```python
from build123d import *

# Parameters (mm, degrees)
F0_W     = 25
F0_H     = 70
F1_DEPTH = 5
F2_W     = 12
F2_H     = 4.5
F3_DEPTH = 14
F4_R     = 2
F5_R     = 5
F6_R     = 1


with BuildPart() as f1:
    # F0 (on Top) → F1 (new body, symmetric)
    with BuildSketch(Plane.XY):
        Rectangle(F0_W, F0_H)
    extrude(amount=F1_DEPTH, both=True)

    # F2 (on face) → F3 (join)
    with BuildSketch(Plane.XZ.offset(35)):
        Rectangle(F2_W, F2_H)
    extrude(amount=F3_DEPTH)

    # F4
    f4_edges = [f1.edges().sort_by_distance(p)[0] for p in [
        (12.5, -35, 0),
        (-12.5, -35, 0),
    ]]
    fillet(f4_edges, radius=F4_R)

    # F5
    f5_edges = [f1.edges().sort_by_distance(p)[0] for p in [
        (12.5, 35, 0),
        (-12.5, 35, 0),
    ]]
    fillet(f5_edges, radius=F5_R)

    # F6
    f6_edges = [f1.edges().sort_by_distance(p)[0] for p in [
        (-12.5, -1.5, 5),
        (-11.035534, 33.535534, 5),
        (-11.914214, -34.414214, 5),
        (0, 35, 5),
        (0, -35, 5),
        (11.035534, 33.535534, 5),
        (11.914214, -34.414214, 5),
        (12.5, -1.5, 5),
        (-12.5, -1.5, -5),
        (-11.035534, 33.535534, -5),
        (-11.914214, -34.414214, -5),
        (0, 35, -5),
        (0, -35, -5),
        (11.035534, 33.535534, -5),
        (11.914214, -34.414214, -5),
        (12.5, -1.5, -5),
    ]]
    fillet(f6_edges, radius=F6_R)


solid = f1.part
```
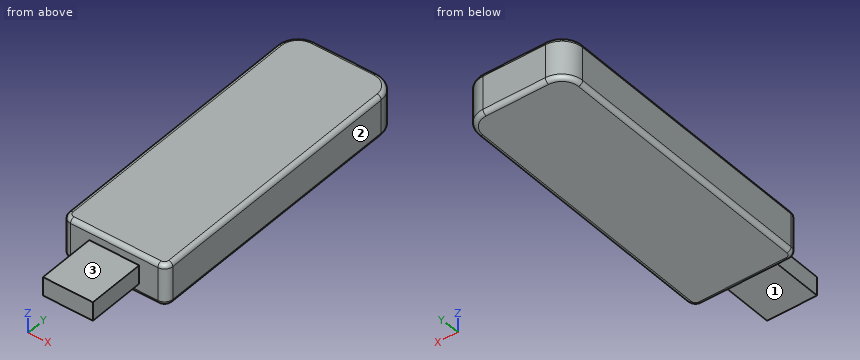
Check sheet for the modelled part. Datum: model origin and axes. Units: mm. Face numbers are marked on the shaded views. A direction names the side the tool comes from. Coordinates: 2 decimals unless noted, no trailing zeros. Loops run counter-clockwise (first coordinate to the right, second up) from the corner with the lowest first, then second, coordinate; pieces in that order, holes last. Notation, with made-up numbers: M -2,72.5 L 40,72.5 A27 ccw 40,101.5 Z; hole C 21,21 d9. An arc over 180 degrees is marked long. Answer as a JSON object with one key per item and string values.
1. Depth check by flat-ended pin: P1, Ø2, axis at y = -39.5, z = -0.5, coming from the +X side; P2, Ø13, axis at x = 2, y = -43, coming from the -Z side; P3, Ø6, axis at x = -1, y = -41, coming from the +Z side. Enter the tip coordinate at first touch or a pass-through.
Outcome:
{"P1": "x = 6", "P2": "z = -2.25", "P3": "z = 2.25"}
2. Access from +Z, -Z, +X, -X, +Y, -Y to the whole of each face (thin tool, end or side, straight path). Record for the marked faces 1, 2 and 3.
Outcome:
{"face 1": "-Z, +X, -X, -Y", "face 2": "+Z, -Z, +X, +Y, -Y", "face 3": "+Z, +X, -X, -Y"}
3. Scan lines: L1, parallel to Y at x = -6.5, z = 1.5; L2, parallel to Z at x = 2, y = -36.5; L3, parallel to X at y = -42.5, z = 1. Record each from-to range of solid material in increasing order. Write a range as from..to.
Outcome:
{"L1": "-35..35", "L2": "-2.25..2.25", "L3": "-6..6"}
4. Sectioned sample at A-A on x = 0. Record the cut outline in (y, z), and give its area (3 significant figures).
Outcome:
{"outline": "M -49,-2.25 L -35,-2.25 L -35,-4 A1 ccw -34,-5 L 34,-5 A1 ccw 35,-4 L 35,4 A1 ccw 34,5 L -34,5 A1 ccw -35,4 L -35,2.25 L -49,2.25 Z", "area": "762 mm²"}
5. Sectioned sample at B-B on z = 3.25. Record the cut outline in (x, y).
Outcome:
{"outline": "M -12.5,-33 A2 ccw -10.5,-35 L 10.5,-35 A2 ccw 12.5,-33 L 12.5,30 A5 ccw 7.5,35 L -7.5,35 A5 ccw -12.5,30 Z"}
6. Sectioned sample at C-C on z = -1. Record the cut outline in (x, y), and give its area (3 significant figures).
Outcome:
{"outline": "M -12.5,-33 A2 ccw -10.5,-35 L -6,-35 L -6,-49 L 6,-49 L 6,-35 L 10.5,-35 A2 ccw 12.5,-33 L 12.5,30 A5 ccw 7.5,35 L -7.5,35 A5 ccw -12.5,30 Z", "area": "1,910 mm²"}
